Input: part model. Units: mm. Frame: model coordinates. A direction names the side the tool comes from. Give positions to 0.01 mm unless a question says otherwise; leave off trailing zeros. Order: outer loops, then holes, each group sorted by start corner. A loop starts at its lowest first (then second) coordinate and runs counter-clockwise, first axis right, second up. Notation, with made-up numbers: (18.25, -16.5) - (22.25, -16.5) arc R22 cw to (22.25, 0.5) - close; hole circle Ø11 at (5, -1). An arc over 180 degrees is marked (long way). Answer in a Markdown table with one row per item. Add a question column.
1. Mould query, pull axis Y, two halves, no side actions, for faces 1 (the face through (29.86, 54.74, -11.04)), 2 (the face through (130, 48, -29)), 3 (the face through (29.86, 72.44, -30.38)). Classes: released by +Y, released by -Y, zero draft, split by the parting line, or undercut.
2. Section query C-C on z = -52.5. Return loops of the section in (x, y).
3. Access query for faces 4 (the face through (120.14, 54.74, -11.04)), 5 (the face through (30, 40, -43.267)), 6 (the face through (76, 8, 0)), 7 (the face through (110, 48, -28)). Directions: +Z, -Z, +X, -X, +Y, -Y. A direction counts if a zero-diameter tool reaches every point of the face in a straight line with its end or side. Return the directions, or none.
4. Contact query for flat-ended pins moving along their axis: pin 1 (6 mm diameter, centred on x = 120.5, y = 46.5, fed in from -Z); pin 2 (4 mm diameter, centred on x = 87.5, y = 18, fed in from -Z); pin 3 (3 mm diameter, centred on y = 61, z = -41.5, fed in from -X); pin 4 (4 mm diameter, centred on x = 105.5, z = -8.5, fed in from +Y). Output: stop coordinate, or through.
5. Section query D-D on y = 61. Return loops of the section in (x, z).
6. Section query A-A on y = 48.5. Return loops of the section in (x, z), and give its area (3 significant figures).
7. Ray query, line 1 (X direction, y = 22, z = -27.5); line 2 (Y direction, x = 137, z = -52); line 3 (Y direction, x = 31, z = -10). Return the intervals inside material, ascending. Write a range as [from, to].
8. Section query B-B on x = 28. Return loops of the section in (y, z).
```python
from build123d import *

# Parameters (mm, degrees)
BOSS_EXTRUDE1_DEPTH = 75
CUT_EXTRUDE5_DEPTH  = 20
CUT_EXTRUDE6_DEPTH  = 35


with BuildPart() as part:
    # Sketch1 → Boss-Extrude1 (new body)
    with BuildSketch(Plane(origin=(0, 0, 0), x_dir=(0, 0, -1), z_dir=(1, 0, 0))):
        Polygon((0, 0), (60, 0), (60, 15), (43.266704148, 15), (43.266704148, 65), (17.121672742, 80.09484092), (4.621672742, 58.444205825), (17.650132663, 50.922220983), (17.650132663, 15), (0, 15), align=None)
    boss_extrude1 = extrude(amount=BOSS_EXTRUDE1_DEPTH)

    # Sketch6 → Cut-Extrude5 (cut)
    with BuildSketch(Plane.ZY):
        Polygon((-43.266704148, 15), (-17.650132663, 15), (-17.650132663, 50.922220983), (-4.621672742, 58.444205825), (-17.121672742, 80.09484092), (-43.266704148, 65), align=None)
    cut_extrude5 = extrude(amount=-CUT_EXTRUDE5_DEPTH, mode=Mode.SUBTRACT)

    # Sketch7 → Cut-Extrude6 (cut)
    with BuildSketch(Plane(origin=(75, 0, 0), x_dir=(0, 0, -1), z_dir=(1, 0, 0))):
        Polygon((17.650132663, 15), (43.266704148, 15), (43.266704148, 65), (17.121672742, 80.09484092), (4.621672742, 58.444205825), (17.650132663, 50.922220983), align=None)
    cut_extrude6 = extrude(amount=-CUT_EXTRUDE6_DEPTH, mode=Mode.SUBTRACT)

    # Mirror2: Boss-Extrude1, Cut-Extrude5, Cut-Extrude6 across plane
    add(boss_extrude1.mirror(Plane(origin=(75, 0, 0), x_dir=(0, 0, 1), z_dir=(1, 0, 0))))
    add(cut_extrude5.mirror(Plane(origin=(75, 0, 0), x_dir=(0, 0, 1), z_dir=(1, 0, 0))), mode=Mode.SUBTRACT)
    add(cut_extrude6.mirror(Plane(origin=(75, 0, 0), x_dir=(0, 0, 1), z_dir=(1, 0, 0))), mode=Mode.SUBTRACT)


solid = part.part
```
Answer:
| question | item | result |
|---|---|---|
| 1 | face 1 | undercut |
| 1 | face 2 | zero draft |
| 1 | face 3 | released by +Y |
| 2 | outline | (0, 0) - (150, 0) - (150, 15) - (0, 15) - close |
| 3 | face 4 | +Z, +X, -X |
| 3 | face 5 | -Z, +X, -X, +Y |
| 3 | face 6 | +Z, +X, -X, +Y, -Y |
| 3 | face 7 | +Z, -Z, +Y |
| 4 | pin 1 | stops at z = -43.27 |
| 4 | pin 2 | passes through |
| 4 | pin 3 | stops at x = 20 |
| 4 | pin 4 | stops at y = 15 |
| 5 | outline | (20, -43.27) - (40, -43.27) - (40, -6.1) - (20, -6.1) - close; (110, -43.27) - (130, -43.27) - (130, -6.1) - (110, -6.1) - close |
| 6 | outline | (20, -43.27) - (40, -43.27) - (40, -17.65) - (20, -17.65) - close; (110, -43.27) - (130, -43.27) - (130, -17.65) - (110, -17.65) - close |
| 6 | area | 1,020 mm² |
| 7 | line 1 | x = [20, 40], [110, 130] |
| 7 | line 2 | y = [0, 15] |
| 7 | line 3 | y = [0, 15], [55.34, 67.76] |
| 8 | outline | (0, -60) - (15, -60) - (15, -43.27) - (65, -43.27) - (80.09, -17.12) - (58.44, -4.62) - (50.92, -17.65) - (15, -17.65) - (15, 0) - (0, 0) - close |
